from build123d import *

# Parameters (mm, degrees)
SKETCH2_R          = 2
CUT_EXTRUDE1_DEPTH = 112.579568022


with BuildPart() as part:
    # Sketch1 → Revolve1 (revolve)
    with BuildSketch(Plane.XY, mode=Mode.PRIVATE) as revolve1_sk:
        Polygon((72.612826049, 25), (72.612826049, 50), (62.612826049, 50), (62.612826049, 35), (57.612826049, 35), (57.612826049, 32), (27.612826049, 32), (27.612826049, 35), (22.612826049, 35), (22.612826049, 55), (-7.387173951, 55), (-7.387173951, 50), (12.612826049, 50), (12.612826049, 40), (-7.387173951, 40), (-7.387173951, 35), (12.612826049, 35), (12.612826049, 25), align=None)
    revolve(revolve1_sk.sketch.rotate(Axis((-41.889027365, 0, 0), (1, 0, 0)), 90), axis=Axis((-41.889027365, 0, 0), (1, 0, 0)))

    # Sketch2 → Cut-Extrude1 (cut, through all)
    with BuildSketch(Plane(origin=(72.612826049, 0, 0), x_dir=(0, 0, -1), z_dir=(1, 0, 0))):
        with Locations((0, 45)):
            Circle(SKETCH2_R)
        with Locations((26.450336353, 36.405764747)):
            Circle(SKETCH2_R)
        with Locations((42.797543233, 13.905764747)):
            Circle(SKETCH2_R)
        with Locations((42.797543233, -13.905764747)):
            Circle(SKETCH2_R)
        with Locations((26.450336353, -36.405764747)):
            Circle(SKETCH2_R)
        with Locations((0, -45)):
            Circle(SKETCH2_R)
        with Locations((-26.450336353, -36.405764747)):
            Circle(SKETCH2_R)
        with Locations((-42.797543233, -13.905764747)):
            Circle(SKETCH2_R)
        with Locations((-42.797543233, 13.905764747)):
            Circle(SKETCH2_R)
        with Locations((-26.450336353, 36.405764747)):
            Circle(SKETCH2_R)
    extrude(amount=-CUT_EXTRUDE1_DEPTH, mode=Mode.SUBTRACT)


solid = part.part
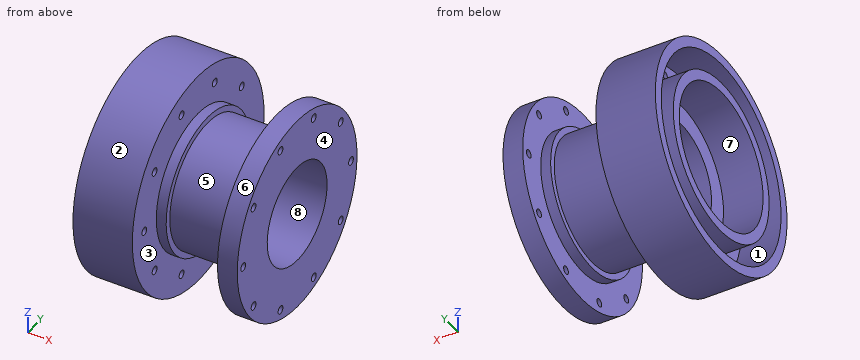
The model under review builds one solid part; all positions refer to its coordinate system, in mm. Face numbers are marked on the shaded views. A direction names the side the tool comes from. Give positions to 0.01 mm unless a question says otherwise; leave off trailing zeros. Write each loop counter-clockwise with the first axis right and the second up, starting at its lowest first coordinate (ties: lowest second). Pieces come first, ordered by that corner, then holes. Notation, with made-up numbers: M 85.25,51 L 108.25,51 A21 ccw 108.25,66 Z; hole C -39.75,32.5 d1. An arc over 180 degrees is marked long. One line per question, with ' | ' between items. Start each with the question number.
Item 1: Draft analysis for pull direction Z (two halves, no side actions). For the marked faces 1, 2 and 3, state which applies: released by +Z, released by -Z, zero draft, split by the parting line, or undercut.
Item 2: We need section C-C on x = 40. Write out the cut boundary in (y, z).
Item 3: We need section D-D on z = -47. Write out the cut boundary in (x, y).
Item 4: For pin 1 (3 mm diameter, centred on y = -38.5, z = -17, fed in from -X); pin 2 (12 mm diameter, centred on x = 9.5, z = -22.5, fed in from +Y); pin 3 (8 mm diameter, centred on x = 3, y = 32, fed in from -Z), all flat-tipped, find the tip position at first contact; note any pin that passes through.
Item 5: For the marked faces 4, 5, 6, 7 and 8, list the 3-axis set-ups (+Z, -Z, +X, -X, +Y, -Y) from which the entire face can be reached by the end or side of a thin tool; tool diameter is ignored.
Item 6: Wall thickness on line 1 (Z direction, x = 10, y = -1); line 2 (Y direction, x = 0.5, z = -23.5); line 3 (Z direction, x = 9, y = 18.5): over which ranges is each line inside the solid? List them lowest first. Write a range as from..to.
Item 7: We need section B-B on z = 0. Give the number of separate pieces and of enclosed holes in the cut face, plus the area to 3 significant figures.
Item 8: We need section A-A on y = -45. Write out the cut boundary in (x, z), plus the area to 3 significant figures.
Results found:
1) face 1: undercut | face 2: split by the parting line | face 3: zero draft
2) outline: C 0,0 d64; hole C 0,0 d50
3) outline: M -7.39,-28.57 L 22.61,-28.57 L 22.61,28.57 L -7.39,28.57 L -7.39,17.06 L 12.61,17.06 L 12.61,-17.06 L -7.39,-17.06 Z; M 62.61,-17.06 L 72.61,-17.06 L 72.61,17.06 L 62.61,17.06 Z
4) pin 1: stops at x = 12.61 | pin 2: stops at y = 52.47 | pin 3: stops at z = -47.34
5) face 4: +Z, -Z, +X, +Y, -Y | face 5: none | face 6: +X | face 7: -X | face 8: +X, -X
6) line 1: z = -54.99..-49.99, -39.99..-34.99, 34.99..39.99, 49.99..54.99 | line 2: y = -49.73..-44.13, -32.37..-25.94, 25.94..32.37, 44.13..49.73 | line 3: z = -51.8..-46.45, -35.46..-29.71, 29.71..35.46, 46.45..51.8
7) separate pieces: 6 | enclosed holes: 0 | area: 1,960 mm2
8) outline: M -7.39,-31.62 L 22.61,-31.62 L 22.61,-2 L 12.61,-2 L 12.61,-21.79 L -7.39,-21.79 Z; M -7.39,21.79 L 12.61,21.79 L 12.61,2 L 22.61,2 L 22.61,31.62 L -7.39,31.62 Z; M 62.61,-21.79 L 72.61,-21.79 L 72.61,-2 L 62.61,-2 Z; M 62.61,2 L 72.61,2 L 72.61,21.79 L 62.61,21.79 Z | area: 1,380 mm2
